```python
from build123d import *

# Parameters (mm, degrees)
SKETCH1_W           = 70
SKETCH1_H           = 10
BOSS_EXTRUDE1_DEPTH = 5
FILLET1_R           = 5
SKETCH2_R           = 2.9
BOSS_EXTRUDE2_DEPTH = 15
SKETCH3_R           = 2.9
BOSS_EXTRUDE3_DEPTH = 35


with BuildPart() as part:
    # Sketch1 → Boss-Extrude1 (new body)
    with BuildSketch(Plane(origin=(0, 0, 0), x_dir=(1, 0, 0), z_dir=(0, 1, 0))):
        with Locations((35, 5)):
            Rectangle(SKETCH1_W, SKETCH1_H)
    extrude(amount=BOSS_EXTRUDE1_DEPTH)

    # Fillet1
    fillet1_edges = [part.edges().sort_by_distance(p)[0] for p in [
        (70, 2.5, -10),
        (70, 2.5, 0),
        (0, 2.5, -10),
        (0, 2.5, 0),
    ]]
    fillet(fillet1_edges, radius=FILLET1_R - 0.0001)  # a hair under: the kernel refuses the full size

    # Sketch2 → Boss-Extrude2 (add)
    with BuildSketch(Plane.XZ):
        with Locations(Location((5, -5, 0), (0, 0, 270))):
            Circle(SKETCH2_R)
    extrude(amount=BOSS_EXTRUDE2_DEPTH)

    # Sketch3 → Boss-Extrude3 (add)
    with BuildSketch(Plane(origin=(0, 5, 0), x_dir=(1, 0, 0), z_dir=(0, 1, 0))):
        with Locations(Location((65, 5, 0), (0, 0, 270))):
            Circle(SKETCH3_R)
    extrude(amount=BOSS_EXTRUDE3_DEPTH)


solid = part.part
```
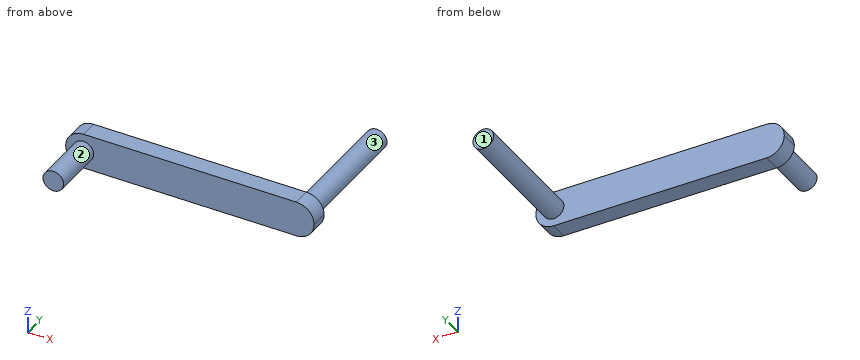
Work out the finished part from the listing and answer in its coordinate system (mm). Face numbers are marked on the shaded views. A direction names the side the tool comes from. Round coordinates to 2 decimals unless told otherwise and drop trailing zeros. Write each loop counter-clockwise with the first axis right and the second up, starting at its lowest first coordinate (ties: lowest second). Pieces come first, ordered by that corner, then holes. Notation, with made-up numbers: (27, 7.25) -> (66, 7.25) arc R37 cw to (66, 43.25) -> close; hole circle Ø2 at (20, 37). An arc over 180 degrees is marked (long way). Write each question's results on one line, items separated by ' | '.
Q1. Flat-ended cylindrical pins translate along their axes: P1, Ø5, axis at x = 44, z = -3.5, coming from the +Y side; P2, Ø6, axis at y = 26.5, z = -7, coming from the -X side. Find the tip coordinate at first contact, or state that the pin passes through.
Data:
P1: y = 5 | P2: x = 62.1
Q2. Section C-C, the plane x = 36 is taken. Write down the section's boundary in (y, z), then the cut area to 3 significant figures.
Data:
outline: (0, -10) -> (5, -10) -> (5, 0) -> (0, 0) -> close | area: 50.0 mm^2
Q3. Straight lines are drawn through the part: line 1 along Y through (x, z) = (43, -5.75); line 2 along Y through (x, z) = (66, -2.5); line 3 along Z through (x, y) = (4, 0.5). For each, find the intervals that lie inside material, in ascending order. Write a range as [from, to].
Data:
line 1: [0, 5] | line 2: [0, 40] | line 3: [-9.9, -0.1]
Q4. Which of the six approach directions +Z, -Z, +X, -X, +Y, -Y give full straight-line access (tool end or side, diameter ignored) to the marked faces 1, 2 and 3?
Data:
face 1: +Z, -Z, +X, -X, +Y | face 2: -Y | face 3: +Y
Q5. Section D-D, the plane y = 9.5 is taken. Write down the section's boundary in (x, z), then the cut area to 3 significant figures.
Data:
outline: circle Ø5.8 at (65, -5) | area: 26.4 mm^2
Q6. Section B-B, the plane z = -6.5 is taken. Write down the section's boundary in (x, y).
Data:
outline: (0.23, 0) -> (2.52, 0) -> (2.52, -15) -> (7.48, -15) -> (7.48, 0) -> (69.77, 0) -> (69.77, 5) -> (67.48, 5) -> (67.48, 40) -> (62.52, 40) -> (62.52, 5) -> (0.23, 5) -> close
